```python
from build123d import *

# Parameters (mm, degrees)
CROQUIS1_W              = 355
CROQUIS1_H              = 443
SALIENTE_EXTRUIR1_DEPTH = 89
CROQUIS2_W              = 482.6
CROQUIS2_H              = 89
SALIENTE_EXTRUIR2_DEPTH = 2


with BuildPart() as part:
    # Croquis1 → Saliente-Extruir1 (new body)
    with BuildSketch(Plane(origin=(0, 0, 0), x_dir=(1, 0, 0), z_dir=(0, 1, 0))):
        Rectangle(CROQUIS1_W, CROQUIS1_H)
    extrude(amount=SALIENTE_EXTRUIR1_DEPTH)

    # Croquis2 → Saliente-Extruir2 (add)
    with BuildSketch(Plane.ZY.offset(177.5)):
        with Locations((0, 44.5)):
            Rectangle(CROQUIS2_W, CROQUIS2_H)
        with BuildLine():
            Line((-233.06, 68.5), (-232.06, 68.5))
            ThreePointArc((-232.06, 68.5), (-228.06, 64.5), (-232.06, 60.5))
            Line((-232.06, 60.5), (-233.06, 60.5))
            ThreePointArc((-233.06, 60.5), (-237.06, 64.5), (-233.06, 68.5))
        make_face(mode=Mode.SUBTRACT)
        with BuildLine():
            Line((-233.06, 20.5), (-232.06, 20.5))
            ThreePointArc((-232.06, 20.5), (-228.06, 24.5), (-232.06, 28.5))
            Line((-232.06, 28.5), (-233.06, 28.5))
            ThreePointArc((-233.06, 28.5), (-237.06, 24.5), (-233.06, 20.5))
        make_face(mode=Mode.SUBTRACT)
        with BuildLine():
            Line((233.06, 68.5), (232.06, 68.5))
            ThreePointArc((232.06, 68.5), (228.06, 64.5), (232.06, 60.5))
            Line((232.06, 60.5), (233.06, 60.5))
            ThreePointArc((233.06, 60.5), (237.06, 64.5), (233.06, 68.5))
        make_face(mode=Mode.SUBTRACT)
        with BuildLine():
            Line((233.06, 20.5), (232.06, 20.5))
            ThreePointArc((232.06, 20.5), (228.06, 24.5), (232.06, 28.5))
            Line((232.06, 28.5), (233.06, 28.5))
            ThreePointArc((233.06, 28.5), (237.06, 24.5), (233.06, 20.5))
        make_face(mode=Mode.SUBTRACT)
    extrude(amount=-SALIENTE_EXTRUIR2_DEPTH)


solid = part.part
```
Here's how the part is built. I have some questions about the finished solid (model axes, mm). A direction names the side the tool comes from. Give positions to 0.01 mm unless a question says otherwise; leave off trailing zeros. Order: outer loops, then holes, each group sorted by start corner. A loop starts at its lowest first (then second) coordinate and runs counter-clockwise, first axis right, second up. Notation, with made-up numbers: M 14,78.5 L 42,78.5 A9 ccw 42,86.5 Z; hole C -25,84.5 d11. An arc over 180 degrees is marked long. Use a Markdown table: item, result. Add a question column.
1. I need wall thicknesses on probe 1 along Z at (x, y) = (157, 59.5). Which ranges of the line are inside material? Lowest first, please. Write a range as from..to.
2. For pin 1 Ø5 at (x, y) = (-125.5, 63.5) entering from +Z; pin 2 Ø10 at (y, z) = (46, 229) entering from +X, each with a flat end and sliding along its axis, tell me the tip position at first contact or that it passes through.
3. On a 3-axis mill with a long thin cutter (end or side, diameter ignored), from which of +Z, -Z, +X, -X, +Y, -Y can I reach the whole of each face in a straight line? I mean faces 1 (the flat face through (-1, 44, -221.5)), 2 (the flat face through (-175.5, 45, 231)), 3 (the flat face through (-2, 89, -3)). Say none if no direction works.
4. Suppose I cut it at A-A (x = 114). List the corners of the cut face in (y, z) for me, and give its area (3 significant figures).
Results list:
| question | item | result |
|---|---|---|
| 1 | probe 1 | z = -221.5..221.5 |
| 2 | pin 1 | stops at z = 221.5 |
| 2 | pin 2 | stops at x = -175.5 |
| 3 | face 1 | -Z, +X, +Y, -Y |
| 3 | face 2 | +Z, +X, +Y, -Y |
| 3 | face 3 | +Z, -Z, +X, -X, +Y |
| 4 | outline | M 0,-221.5 L 89,-221.5 L 89,221.5 L 0,221.5 Z |
| 4 | area | 39,400 mm² |
